Autodesk Inventor part; units mm, degrees
ref_plane "YZ Plane" through (0, 0, 0) normal (1, 0, 0) x (0, 1, 0)
ref_plane "XZ Plane" through (0, 0, 0) normal (0, 1, 0) x (-1, 0, 0)
ref_plane "XY Plane" through (0, 0, 0) normal (0, 0, 1) x (1, 0, 0)
ref_plane "Work Plane1" through (-72.8386, -105.7169, -152.268) normal (1, 0, 0) x (0, 1, 0)
sketch "Sketch1" plane through (-72.8386, -105.7169, -152.268) normal (1, 0, 0) x (0, 1, 0)
  line L0 (-41.2196, 6.35) -> (64.7019, 6.35)
  circle A0 centre (0, 6.35) radius 2.1844
  line L1 (-12.7, -5.2578) -> (-12.7, 56.2102)
  line L2 (-24.13, 6.35) -> (-24.13, -171.3455)
  line L3 (-22.1107, -175.9896) -> (-9.7415, -187.5241)
  line L4 (-5.4108, -189.23) -> (23.8328, -189.23)
  circle A1 centre (52.4757, -106.725) radius 2.1844
  line L5 (12.7, 56.2102) -> (12.7, -5.2578)
  circle A2 centre (52.4757, -106.725) radius 7.62
  line L6 (2.3114, -184.15) -> (10.3188, -184.15)
  line L7 (-12.7, -184.15) -> (-12.7, -134.2898)
  line L8 (59.5652, -109.5185) -> (29.7407, -185.2079)
  line L9 (-24.13, 5.842) -> (67.0388, 5.842)
  line L10 (59.3372, -103.4107) -> (15.2284, -12.0924)
  line L11 (12.7, -1.0449) -> (12.7, 5.842)
  circle A3 centre (21.8059, -177.8) radius 2.1844
  circle A4 centre (21.8059, -165.1) radius 2.1844
  circle A5 centre (-6.35, -76.2) radius 2.1844
  circle A6 centre (-6.35, -76.2) radius 20.32
  line L12 (-24.13, -50.8) -> (-24.13, -63.5) construction
  line L13 (-24.13, -63.5) -> (-36.83, -76.2) construction
  line L14 (-36.83, -76.2) -> (-24.13, -88.9) construction
  line L15 (-24.13, -88.9) -> (-24.13, -101.6) construction
  spline S0 degree 4 poles (-24.13, -50.8) (-24.13, -63.5) (-36.83, -76.2) (-24.13, -88.9) (-24.13, -101.6) knots 1 1 1 1 1 2 2 2 2 2
  arc A7 (12.7, -1.0449) -> (15.2284, -12.0924) centre (38.1, -1.0449) ccw
  arc A8 (23.8328, -189.23) -> (29.7407, -185.2079) centre (23.8328, -182.88) ccw
  arc A9 (-9.7415, -187.5241) -> (-5.4108, -189.23) centre (-5.4108, -182.88) ccw
  arc A10 (-24.13, -171.3455) -> (-22.1107, -175.9896) centre (-17.78, -171.3455) ccw
  circle A11 centre (6.35, -38.1) radius 2.1844
  circle A12 centre (6.35, -38.1) radius 5.08
  circle A13 centre (6.35, -127) radius 2.1844
  circle A14 centre (6.35, -127) radius 5.08
  circle A15 centre (0, -82.55) radius 2.1844
  line L16 (10.3187, 184.15) -> (-10.3187, 184.15)
  circle A16 centre (6.35, -25.4) radius 2.1844
  circle A17 centre (6.35, -12.7) radius 2.1844
  circle A18 centre (6.35, 0) radius 2.1844
  circle A19 centre (-6.35, -177.8) radius 2.1844
  circle A20 centre (0, -6.35) radius 2.1844
  circle A21 centre (0, -19.05) radius 2.1844
  point P0 (105.7169, 152.268)
  point P1 (-7.9121, -189.23)
  point P2 (28.1559, -189.23)
  point P3 (12.7, -6.858)
  point P4 (12.7, -1.0449)
  point P5 (12.7, 5.842)
  point P6 (2.1245, 5.842)
  point P7 (-2.1245, 5.842)
  point P8 (-24.13, -66.3626)
  point P9 (-24.13, -86.0374)
  dimension "d0" = 15.24
  dimension "d1" = 5.08
  dimension "d3" = 11.43
  dimension "d4" = 133
  dimension "d5" = 40.64
  dimension "d6" = 6.35
  dimension "d7" = 36.068
  dimension "d8" = 0.508
  dimension "d9" = 12.7
  dimension "d10" = 12.7
  dimension "d11" = 12.7
  dimension "d12" = 12.7
  dimension "d13" = 12.7
  dimension "d14" = 12.7
  dimension "d15" = 25.4
  dimension "d16" = 6.35
  dimension "d17" = 10.16
  dimension "d18" = 10.16
  dimension "d21" = 12.7
  dimension "d22" = 12.7
  dimension "d23" = 4.3688
  dimension "d24" = 4.3688
extrude "Extrusion1" add sketch "Sketch1" along normal blind 1.5875 contours L9 A0 L5 A7 L10 A2 L8 A8 L4 A9 L3 A10 L2 A6 | L2 A6 S0 | A6 L2 | L2 A6 | A2 | A15 | A16 | A17 | A18
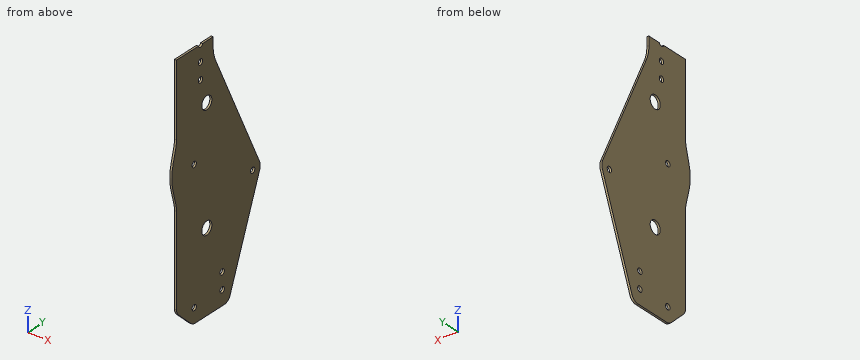
Verification items for the finished model (mm, model axes). Give positions to 0.01 mm unless a question says otherwise; leave off trailing zeros. Write each loop counter-clockwise with the first axis right and the second up, starting at its lowest first coordinate (ties: lowest second). Pieces come first, ordered by that corner, then holes. Notation, with made-up numbers: M -11,-9.75 L 41,-9.75 A18 ccw 41,23.25 Z; hole C -13,55.25 d5. An arc over 180 degrees is marked long. Write item = value, one per line.
(1) Sectioned sample at C-C (y = -88.5). Record the cut outline in (x, z), then the cut area to 3 significant figures.
Found:
outline = M -72.84,-341.5 L -71.25,-341.5 L -71.25,-168.48 L -72.84,-168.48 Z
area = 275 mm2
(2) Material ranges on line 1 (Z direction, x = -72, y = -106); line 2 (Z direction, x = -71.85, y = -110.5); line 3 (Y direction, x = -72.5, z = -319), recorded low to high.
Found:
line_1 = -341.5 to -173.48, -169.15 to -160.78, -156.45 to -148.08
line_2 = -341.5 to -331.59, -328.55 to -229.99, -226.95 to -146.43
line_3 = -129.85 to -85.36, -82.46 to -68.7
(3) Sectioned sample at A-A (x = -71.55). Give the number of separate pieces and of enclosed holes in the cut face, then the cut area to 3 significant figures.
Found:
separate_pieces = 1
enclosed_holes = 9
area = 11,900 mm2
(4) Go/stop test with flat-tipped pins: pin 1 Ø4 at (y, z) = (-105.72, -158.62) entering from +X; pin 2 Ø0.8 at (x, z) = (-72.5, -304.5) entering from -Y. Record where each tip stops, or that it passes through.
Found:
pin_1 = through
pin_2 = -129.85
(5) Sectioned sample at B-B (z = -294.5). Record the cut outline in (x, y).
Found:
outline = M -72.84,-129.85 L -71.25,-129.85 L -71.25,-59.04 L -72.84,-59.04 Z
